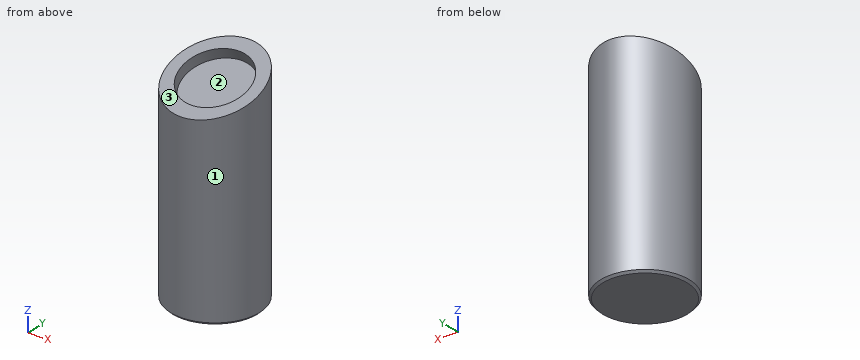
from build123d import *

# Parameters (mm, degrees)
F0_R          = 12.5
F1_DEPTH      = 60
F3_DEPTH      = 12.501
F3_DEPTH_BACK = 12.501
F4_R          = 9.25
F5_DEPTH      = 3
F6_SIZE       = 0.6


with BuildPart() as f1:
    # F0 (on Top) → F1 (new body)
    with BuildSketch(Plane.XY):
        Circle(F0_R)
    extrude(amount=F1_DEPTH)

    # F2 (on Right) → F3 (cut, two sides)
    with BuildSketch(Plane.YZ) as f3_sk:
        Polygon((12.5, 60), (-12.5, 60), (-12.5, 51.156578049), align=None)
    extrude(amount=-F3_DEPTH, mode=Mode.SUBTRACT)
    extrude(f3_sk.sketch, amount=F3_DEPTH_BACK, mode=Mode.SUBTRACT)

    # F4 (on face) → F5 (cut)
    with BuildSketch(Plane(origin=(0, -17.4736202127, 49.3972251624), x_dir=(1, 0, 0), z_dir=(0, -0.3334870921, 0.9427546655))):
        with Locations((0, 18.5346419929)):
            Circle(F4_R)
    extrude(amount=-F5_DEPTH, mode=Mode.SUBTRACT)

    # F6
    f6_edges = [f1.edges().sort_by_distance(p)[0] for p in [
        (-12.5, 0, 0),
    ]]
    chamfer(f6_edges, length=F6_SIZE)


solid = f1.part
Work out the finished part from the listing and answer in its coordinate system (mm). Face numbers are marked on the shaded views. Coordinates: 2 decimals unless noted, no trailing zeros. Loops run counter-clockwise (first coordinate to the right, second up) from the corner with the lowest first, then second, coordinate; pieces in that order, holes last. Notation, with made-up numbers: (20.5, 39) -> (33.5, 39) arc R16 cw to (33.5, 55) -> close; hole circle Ø5 at (-10.75, 19). An arc over 180 degrees is marked (long way). Write each question's results on one line, items separated by ' | '. Start each with the question number.
1) Find section B-B on z = 42. Determine the outline of the cut face in (x, y), then the cut area to 3 significant figures.
2) Find section A-A on x = 0. Determine the outline of the cut face in (y, z).
3) Consider line 1 along X through (y, z) = (8, 56); line 2 along X through (y, z) = (-0.25, 42.5); line 3 along X through (y, z) = (-4.5, 31). Determine where each line is inside the solid, lowest interval first.
4) Flat-ended cylindrical pins translate along their axes: P1, Ø1.5, axis at x = -2.5, z = 48, coming from the +Y side; P2, Ø3, axis at x = -7, z = 8, coming from the -Y side (3 decimals); P3, Ø5, axis at x = -2, y = 8.5, coming from the +Z side. Find the tip coordinate at first contact, or state that the pin passes through.
5) The mould has two halves that part along X. Classify the marked faces 1, 2 and 3: pulls with the +X half, pulls with the -X half, needs draft (parallel to the pull), parting line crosses it, or undercut.
Response values:
1) outline: circle Ø25 at (0, 0) | area: 491 mm^2
2) outline: (-12.5, 0.6) -> (-11.9, 0) -> (11.9, 0) -> (12.5, 0.6) -> (12.5, 60) -> (8.72, 58.66) -> (9.72, 55.83) -> (-7.72, 49.67) -> (-8.72, 52.49) -> (-12.5, 51.16) -> close
3) line 1: x = -9.6 to -5.15, 5.15 to 9.6 | line 2: x = -12.5 to 12.5 | line 3: x = -11.66 to 11.66
4) P1: stops at y = 12.38 | P2: stops at y = -11.225 | P3: stops at z = 59.47
5) face 1: parting line crosses it | face 2: undercut | face 3: needs draft
